```python
from build123d import *

# Parameters (mm, degrees)
F0_W     = 128.1502880156
F0_H     = 99.4144454598
F1_DEPTH = 46.99
F3_W     = 64.353780821
F3_H     = 21.5152939782
F4_DEPTH = 102.7512880156
F5_W     = 41.3016797975
F5_H     = 23.244202137
F6_DEPTH = 167.894
F7_DEPTH = 64.008
F8_DEPTH = 88.138


with BuildPart() as f1:
    # F0 (on Top) → F1 (new body)
    with BuildSketch(Plane.XY):
        with Locations((15.0564964861, 6.8030394614)):
            Rectangle(F0_W, F0_H)
    extrude(amount=F1_DEPTH)

    # F3 (on offset) → F4 (cut, through all)
    with BuildSketch(Plane(origin=(-23.6186475217, 0, 0), x_dir=(0, -1, 0), z_dir=(-1, 0, 0))):
        with Locations((-5.138698034, 26.2697902508)):
            Rectangle(F3_W, F3_H)
    extrude(amount=-F4_DEPTH, mode=Mode.SUBTRACT)

    # F5 (on offset) → F6 (cut)
    with BuildSketch(Plane(origin=(-23.6186475217, 0, 0), x_dir=(0, -1, 0), z_dir=(-1, 0, 0))):
        with Locations((-8.3083617501, 44.8075197637)):
            Rectangle(F5_W, F5_H)
    extrude(amount=-F6_DEPTH, mode=Mode.SUBTRACT)

    # F3 (on offset) → F7 (cut)
    with BuildSketch(Plane(origin=(-23.6186475217, 0, 0), x_dir=(0, -1, 0), z_dir=(-1, 0, 0))):
        with Locations((-5.138698034, 26.2697902508)):
            Rectangle(F3_W, F3_H)
    extrude(amount=F7_DEPTH, mode=Mode.SUBTRACT)

    # F5 (on offset) → F8 (cut)
    with BuildSketch(Plane(origin=(-23.6186475217, 0, 0), x_dir=(0, -1, 0), z_dir=(-1, 0, 0))):
        with Locations((-8.3083617501, 44.8075197637)):
            Rectangle(F5_W, F5_H)
    extrude(amount=F8_DEPTH, mode=Mode.SUBTRACT)


solid = f1.part
```
Geometry check sheet. Reference: the model listing, model coordinates, mm. A direction names the side the tool comes from. Coordinates: 2 decimals unless noted, no trailing zeros. Loops run counter-clockwise (first coordinate to the right, second up) from the corner with the lowest first, then second, coordinate; pieces in that order, holes last.
Item 1: Sectioned sample at C-C, the plane x = -2.5. Record the boundary of the cut face in (y, z).
Item 2: Sectioned sample at D-D, the plane y = 17. Record the boundary of the cut face in (x, z), then the cut area to 3 significant figures.
Item 3: Sectioned sample at A-A, the plane z = 22. Record the boundary of the cut face in (x, y).
Item 4: Go/stop test with a flat-tipped pin: pin 1 Ø10 at (x, y) = (-19.5, 17) entering from +Z. Record where the tip stops, or that it passes through.
Item 5: Thickness scan on line 1 (Z direction, x = -28.5, y = 31.5); line 2 (Y direction, x = -24.5, z = 36); line 3 (Y direction, x = 26, z = 39). Record the ranges inside material, lowest first.
Item 6: Release check for a two-part mould opening along Z. For faces 4 (the face through (14, 43, 46.99)), 5 (the face through (16, 33, 37.027)), 6 (the face through (14, -42.904, 23)) record: released by +Z, released by -Z, zero draft, split by the parting line, or undercut.
Item 7: Sectioned sample at B-B, the plane y = -17. Record the boundary of the cut face in (x, z).
Item 8: Access from +Z, -Z, +X, -X, +Y, -Y to the whole of each face (thin tool, end or side, straight path). Record for faces 1 (the face through (16, 28.959, 42)), 2 (the face through (14, 56.51, 23)), 3 (the face through (16, -20, 37.027)).
Check result:
1. outline: (-42.9, 0) - (56.51, 0) - (56.51, 46.99) - (28.96, 46.99) - (28.96, 37.03) - (37.32, 37.03) - (37.32, 15.51) - (-27.04, 15.51) - (-27.04, 37.03) - (-12.34, 37.03) - (-12.34, 46.99) - (-42.9, 46.99) - close
2. outline: (-49.02, 0) - (79.13, 0) - (79.13, 15.51) - (-49.02, 15.51) - close
2. area: 1,990 mm2
3. outline: (-49.02, -42.9) - (79.13, -42.9) - (79.13, -27.04) - (-49.02, -27.04) - close; (-49.02, 37.32) - (79.13, 37.32) - (79.13, 56.51) - (-49.02, 56.51) - close
4. pin 1: stops at z = 15.51
5. line 1: z = 0 to 15.51, 37.03 to 46.99
5. line 2: y = -42.9 to -27.04, 37.32 to 56.51
5. line 3: y = -42.9 to -12.34, 28.96 to 56.51
6. face 4: released by +Z
6. face 5: undercut
6. face 6: zero draft
7. outline: (-49.02, 0) - (79.13, 0) - (79.13, 15.51) - (-49.02, 15.51) - close; (-49.02, 37.03) - (79.13, 37.03) - (79.13, 46.99) - (-49.02, 46.99) - close
8. face 1: +Z, +X, -X
8. face 2: +Z, -Z, +X, -X, +Y
8. face 3: +X, -X
